```python
from build123d import *

# Parameters (mm, degrees)
SKETCH_1_R          = 3.264424224
EXTRUDE_1_DEPTH     = 50
SKETCH_2_OUTSIDE_W  = 31.412
SKETCH_2_OUTSIDE_H  = 34.196
SKETCH_2_OUTSIDE_R  = 6.567936001
CUT_EXTRUDE_1_DEPTH = 20
SKETCH_3_R          = 5
CUT_EXTRUDE_2_DEPTH = 5


with BuildPart() as part:
    # Эскиз1 → Бобышка-Вытянуть1 (new body)
    with BuildSketch(Plane(origin=(0, 0, 0), x_dir=(1, 0, 0), z_dir=(0, 1, 0))):
        Polygon((0, 10.392304845), (-9, 5.196152423), (-9, -5.196152423), (0, -10.392304845), (9, -5.196152423), (9, 5.196152423), align=None)
        Circle(SKETCH_1_R, mode=Mode.SUBTRACT)
    extrude(amount=EXTRUDE_1_DEPTH)

    # Эскиз2 outside → Вырез-Вытянуть1 (cut)
    with BuildSketch(Plane.XZ):
        Rectangle(SKETCH_2_OUTSIDE_W, SKETCH_2_OUTSIDE_H)
        Circle(SKETCH_2_OUTSIDE_R, mode=Mode.SUBTRACT)
    extrude(amount=-CUT_EXTRUDE_1_DEPTH, mode=Mode.SUBTRACT)

    # Эскиз3 → Вырез-Вытянуть2 (cut)
    with BuildSketch(Plane(origin=(0, 50, 0), x_dir=(1, 0, 0), z_dir=(0, 1, 0))):
        Circle(SKETCH_3_R)
    extrude(amount=-CUT_EXTRUDE_2_DEPTH, mode=Mode.SUBTRACT)


solid = part.part
```
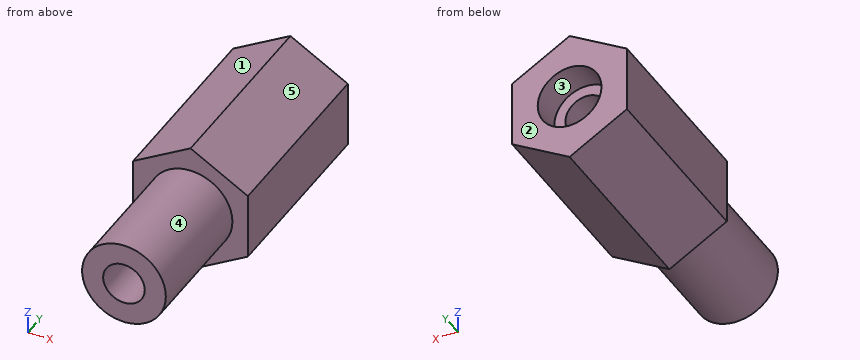
Source: CAD feature listing. Evaluate the final solid. Frame: model axes, mm. Face numbers are marked on the shaded views. A direction names the side the tool comes from. Coordinates: 2 decimals unless noted, no trailing zeros. Loops run counter-clockwise (first coordinate to the right, second up) from the corner with the lowest first, then second, coordinate; pieces in that order, holes last. Notation, with made-up numbers: M 6,70.25 L 35,70.25 A11 cw 35,82.25 Z; hole C 21.25,21.25 d10. An arc over 180 degrees is marked long. Use a Markdown table: item, result. Add a question column.
Q1. Material intervals for L1, parallel to X at y = 48.6, z = 0; L2, parallel to Z at x = 0, y = 48.75; L3, parallel to X at y = 28.5, z = 0, sorted ascending.
Q2. Section query B-B, the plane z = 0. Return loops of the section in (x, y), and give its area (3 significant figures).
Q3. Section query D-D, the plane x = -6. Return loops of the section in (y, z), and give its area (3 significant figures).
Q4. First-contact query: pin 1 (10 mm diameter, centred on x = -5.5, y = 36.5, fed in from +Z). Flat tip, straight axial feed; report the tip coordinate or a pass-through.
Q5. Draft query along X for the marked faces 1, 2 and 3. Return one class per face: pulls with the +X half, pulls with the -X half, needs draft (parallel to the pull), parting line crosses it, or undercut.
Q6. Section query A-A, the plane y = 44.5. Return loops of the section in (x, z).
Q7. Section query C-C, the plane z = -4.5. Return loops of the section in (x, y).
Q8. Access query for the marked faces 4 and 5. Directions: +Z, -Z, +X, -X, +Y, -Y. A direction counts if a zero-diameter tool reaches every point of the face in a straight line with its end or side. Return the directions, or none.
Result:
| question | item | result |
|---|---|---|
| 1 | L1 | x = -9 to -5, 5 to 9 |
| 1 | L2 | z = -10.39 to -5, 5 to 10.39 |
| 1 | L3 | x = -9 to -3.26, 3.26 to 9 |
| 2 | outline | M -9,20 L -6.57,20 L -6.57,0 L -3.26,0 L -3.26,45 L -5,45 L -5,50 L -9,50 Z; M 3.26,0 L 6.57,0 L 6.57,20 L 9,20 L 9,50 L 5,50 L 5,45 L 3.26,45 Z |
| 2 | area | 459 mm2 |
| 3 | outline | M 0,-2.67 L 20,-2.67 L 20,-6.93 L 50,-6.93 L 50,6.93 L 20,6.93 L 20,2.67 L 0,2.67 Z |
| 3 | area | 523 mm2 |
| 4 | pin 1 | stops at z = 10.1 |
| 5 | face 1 | pulls with the -X half |
| 5 | face 2 | needs draft |
| 5 | face 3 | undercut |
| 6 | outline | M -9,-5.2 L 0,-10.39 L 9,-5.2 L 9,5.2 L 0,10.39 L -9,5.2 Z; hole C 0,0 d6.53 |
| 7 | outline | M -9,20 L -4.78,20 L -4.78,0 L 4.78,0 L 4.78,20 L 9,20 L 9,50 L 2.18,50 L 2.18,45 L -2.18,45 L -2.18,50 L -9,50 Z |
| 8 | face 4 | -Y |
| 8 | face 5 | +Z, +X, +Y, -Y |
